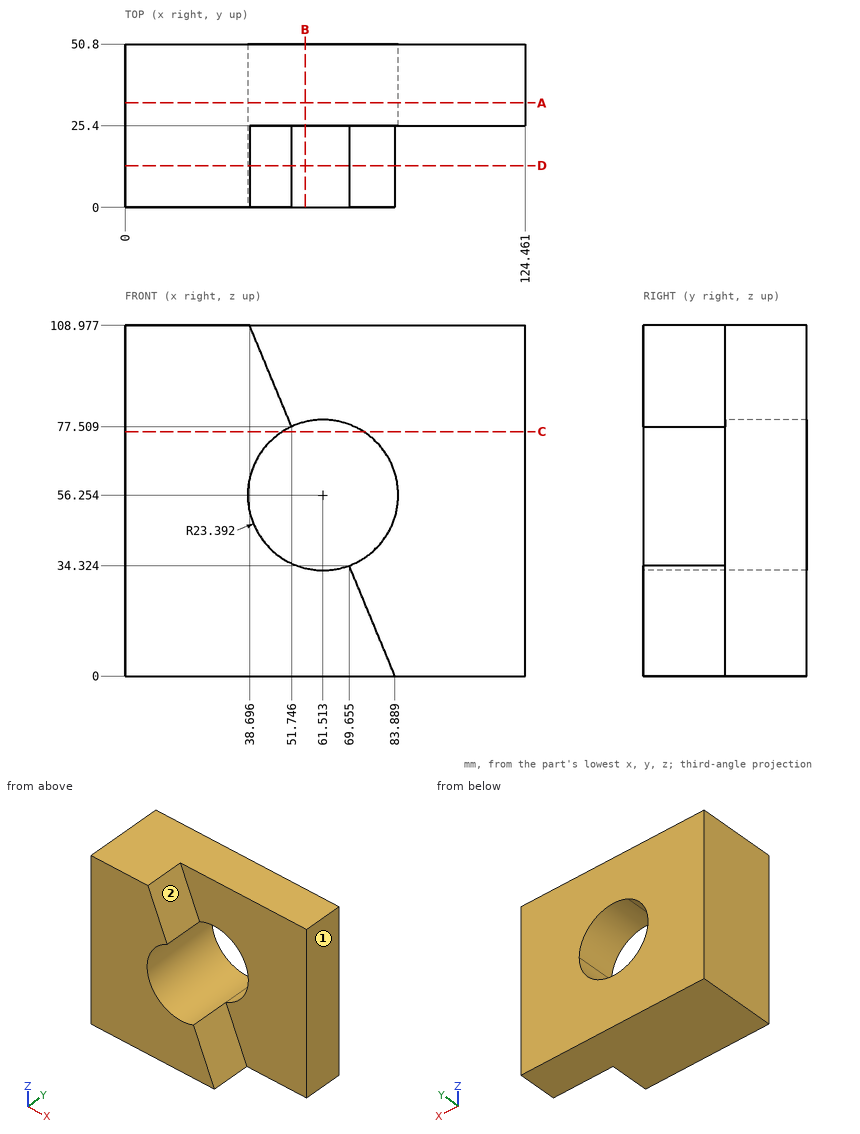
Verification items for this drawing (mm, ordinates from the low corner). A direction names the side the tool comes from. Coordinates: 2 decimals unless noted, no trailing zeros. Write each loop counter-clockwise with the first axis right and the second up, starting at its lowest first coordinate (ties: lowest second). Pieces come first, ordered by that corner, then holes. Notation, with made-up numbers: M -34.5,-4 L -5.5,-4 A14 ccw -5.5,16 Z; hole C 88,61 d7. An arc over 180 degrees is marked long. Use one line per item in the form item = value. Start each with the question number.
1) Section check D-D on y = 13. Enter the section's corners in (x, z) (1 decimal), and give its area (3 significant figures).
2) Section check A-A on y = 32.5. Enter the section's corners in (x, z) (1 decimal).
3) Thickness scan on probe 1 along Z at (x, y) = (60.5, 27) (1 decimal); probe 2 along Y at (x, z) = (93, 43.5); probe 3 along Z at (x, y) = (69, 31) (1 decimal). Record the ranges inside material, lowest first. Write a range as from..to.
4) Go/stop test with flat-tipped pins: pin 1 Ø10 at (x, y) = (109, 19) entering from -Z; pin 2 Ø12 at (x, y) = (88.5, 9) entering from +Z. Record where each tip stops, or that it passes through.
5) Section check B-B on x = 56. Enter the section's corners in (y, z), and give its area (3 significant figures).
6) Set-up check for the marked faces 1 and 2: record each of +Z, -Z, +X, -X, +Y, -Y from which the full face is reachable in a straight line by a thin tool's end or side.
7) Section check C-C on z = 76. Enter the section's corners in (x, y) (1 decimal).
Responses:
q1.outline = M 0,0 L 83.9,0 L 69.7,34.3 A23.4 cw 51.7,77.5 L 38.7,109 L 0,109 Z
q1.area = 5,860 mm2
q2.outline = M 0,0 L 124.5,0 L 124.5,109 L 0,109 Z; hole C 61.5,56.3 d46.8
q3.probe_1 = 0..32.9, 79.6..109
q3.probe_2 = 25.4..50.8
q3.probe_3 = 0..34.1, 78.4..109
q4.pin_1 = through
q4.pin_2 = 3.35
q5.outline = M 0,0 L 50.8,0 L 50.8,33.52 L 0,33.52 Z; M 25.4,78.99 L 50.8,78.99 L 50.8,108.98 L 25.4,108.98 Z
q5.area = 2,460 mm2
q6.face_1 = +Z, -Z, +X, +Y, -Y
q6.face_2 = +Z, +X, -Y
q7.outline = M 0,0 L 49,0 L 49,50.8 L 0,50.8 Z; M 74.1,25.4 L 124.5,25.4 L 124.5,50.8 L 74.1,50.8 Z
